Model file for the job. Use its own axes, mm. A direction names the side the tool comes from. Give positions to 0.01 mm unless a question says otherwise; leave off trailing zeros. Write each loop counter-clockwise with the first axis right and the second up, starting at its lowest first coordinate (ties: lowest second). Pieces come first, ordered by that corner, then holes.
```python
from build123d import *

# Parameters (mm, degrees)
FILLET1_R = 2.5
FILLET2_R = 0.5


with BuildPart() as part:
    # Sketch1 → Revolve1 (revolve)
    with BuildSketch(Plane(origin=(0, 0, 0), x_dir=(1, 0, 0), z_dir=(0, 1, 0))):
        Polygon((0, 19), (10.125, 19), (10.125, 20), (12.125, 20), (12.125, 25.5), (0, 25.5), align=None)
    revolve1 = revolve(axis=Axis((0, 0, 0), (1, 0, 0)))

    # Mirror1: Revolve1 across plane
    add(revolve1.mirror(Plane(origin=(0, 0, 0), x_dir=(0, 0, 1), z_dir=(1, 0, 0))))

    # Fillet1
    fillet1_edges = [part.edges().sort_by_distance(p)[0] for p in [
        (-12.125, 0, 25.5),
        (12.125, 0, 25.5),
    ]]
    fillet(fillet1_edges, radius=FILLET1_R)

    # Fillet2
    fillet2_edges = [part.edges().sort_by_distance(p)[0] for p in [
        (-12.125, 0, 20),
        (12.125, 0, 20),
    ]]
    fillet(fillet2_edges, radius=FILLET2_R)


solid = part.part
```
1. Which spindle directions (+Z, -Z, +X, -X, +Y, -Y) get a long thin tool onto all of the face, cutting with end or side? Do faces 1 (the flat face through (-10.125, -7, 18)), 2 (the flat face through (-12.125, -2, -21)), 3 (the cylindrical face through (10.886, -19.524, 4.336)). Say none if no direction does.
Calculated:
face 1: -X
face 2: +Z, -Z, -X, +Y, -Y
face 3: +X
2. Pull direction Y, two halves, no side cores. Call faces 4 (the cylindrical face through (-10.886, -19.524, 4.336)), 5 (the flat face through (10.125, -7, 18)), 6 (the flat face through (12.125, -2, -21)), 7 (the cylindrical face through (0.1, -24.9, 5.5)): +Y half, -Y half, draft (parallel to the pull), parting line (faces both ways), or undercut.
Calculated:
face 4: undercut
face 5: undercut
face 6: draft
face 7: parting line
3. Probe probe 1 along Y at (x, z) = (-10.5, 15); probe 2 along Z at (x, y) = (4.5, 0.5); probe 3 along Z at (x, y) = (0, -17). List the from-to ranges inside material, lowest first.
Calculated:
probe 1: y = -20.43 to -13.23, 13.23 to 20.43
probe 2: z = -25.5 to -18.99, 18.99 to 25.5
probe 3: z = -19.01 to -8.49, 8.49 to 19.01
4. Pin check, flat tips, straight feed: P1, Ø5, axis at x = -1.5, y = -17.5, coming from the -Z side; P2, Ø1, axis at x = 9, y = 17.5, coming from the +Z side; P3, Ø2, axis at x = -5.5, z = 12, coming from the +Y side; P4, Ø2, axis at y = 19, z = 14, coming from the +X side (3 decimals). Stop position of each tip, or through.
Calculated:
P1: stops at z = -20.62
P2: stops at z = 19.01
P3: stops at y = 23.01
P4: stops at x = 12.125
5. Slice it at A-A, the plane z = 0. Write the cut outline in (x, y) (3 decimals).
Calculated:
outline: (-12.125, -23) arc R2.5 ccw to (-9.625, -25.5) - (9.625, -25.5) arc R2.5 ccw to (12.125, -23) - (12.125, -20.5) arc R0.5 ccw to (11.625, -20) - (10.125, -20) - (10.125, -19) - (-10.125, -19) - (-10.125, -20) - (-11.625, -20) arc R0.5 ccw to (-12.125, -20.5) - close; (-12.125, 20.5) arc R0.5 ccw to (-11.625, 20) - (-10.125, 20) - (-10.125, 19) - (10.125, 19) - (10.125, 20) - (11.625, 20) arc R0.5 ccw to (12.125, 20.5) - (12.125, 23) arc R2.5 ccw to (9.625, 25.5) - (-9.625, 25.5) arc R2.5 ccw to (-12.125, 23) - close
6. Slice it at C-C, the plane x = 0.75. Write the cut outline in (y, z), and give its area (3 significant figures).
Calculated:
outline: circle Ø51 at (0, 0); hole circle Ø38 at (0, 0)
area: 909 mm2
